The listing builds one solid part. Answer for the finished solid, in the listing's coordinates (mm). Face numbers are marked on the shaded views. A direction names the side the tool comes from. Round coordinates to 2 decimals unless told otherwise and drop trailing zeros. Write each loop counter-clockwise with the first axis right and the second up, starting at its lowest first coordinate (ties: lowest second). Pieces come first, ordered by that corner, then holes.
Item 1: A tool of negligible diameter and unlimited length cuts with its end or side. For the marked faces 1, 2 and 3, from which of +Z, -Z, +X, -X, +Y, -Y can it reach the whole face along a straight path? Write none if from no direction.
Item 2: Find section C-C on y = 6.75. Give the vertices of the cut face in (x, z).
Item 3: Find section B-B on z = -14.75. Give the vertices of the cut face in (x, y).
Item 4: This flat-tipped pin is pushed along its axis until it touches: pin 1 (0.5 mm diameter, centred on x = 0, y = 6.5, fed in from +Z). Where does it stop, or does it pass through?
Item 5: Find section A-A on x = -3. Give the vertices of the cut face in (y, z), then the cut area to 3 significant figures.
Item 6: Find the intervals of material crossed by probe 1 along X at (y, z) = (7, -16); probe 2 along Z at (x, y) = (2, 6.3); probe 3 along Z at (x, y) = (-3, 5.8), in increasing order.
Item 7: Find section D-D on x = -0.25. Give the vertices of the cut face in (y, z), then the cut area to 3 significant figures.
```python
from build123d import *

# Parameters (mm, degrees)
SKETCH1_W           = 80
SKETCH1_H           = 80
SKETCH1_R           = 5
SKETCH1_W_2         = 50
SKETCH1_H_2         = 20
BOSS_EXTRUDE2_DEPTH = 3
BOSS_EXTRUDE3_DEPTH = 20
SCALE2_SCALE        = 0.1


with BuildPart() as part:
    # Sketch1 → Boss-Extrude2 (new body)
    # profile 1 of 2: a face of its own
    with BuildSketch(Plane(origin=(0, 0, 0), x_dir=(1, 0, 0), z_dir=(0, 1, 0))):
        Rectangle(SKETCH1_W, SKETCH1_H)
        with Locations(Location((-30, 30, 0), (0, 0, 90))):
            Circle(SKETCH1_R, mode=Mode.SUBTRACT)
        with Locations(Location((30, 30, 0), (0, 0, 90))):
            Circle(SKETCH1_R, mode=Mode.SUBTRACT)
    # profile 2 of 2: a face of its own
    with BuildSketch(Plane(origin=(0, 0, 0), x_dir=(1, 0, 0), z_dir=(0, 1, 0))):
        with Locations((0, 30)):
            Rectangle(SKETCH1_W_2, SKETCH1_H_2)
    extrude(amount=BOSS_EXTRUDE2_DEPTH)

    # Sketch1_5 → Boss-Extrude3 (add)
    with BuildSketch(Plane(origin=(0, 0, 0), x_dir=(1, 0, 0), z_dir=(0, 1, 0))):
        Polygon((25, 40), (-25, 40), (-25, 30), (-25, 20), (25, 20), (25, 30), align=None)
    extrude(amount=BOSS_EXTRUDE3_DEPTH)


with BuildPart() as part_1:
    # Scale2: scaled about (0, 6.258071502, -13.878534205)
    add(part.part.scale(SCALE2_SCALE).moved(Location((0, 5.632264352, -12.490680785))))


solid = part_1.part
```
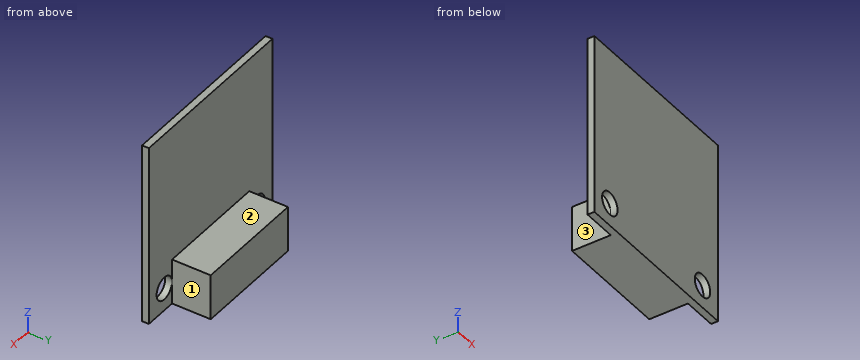
Check values:
1. face 1: +Z, -Z, +X, +Y
1. face 2: +Z, +X, -X, +Y
1. face 3: +Z, -Z, -X, +Y
2. outline: (-2.5, -16.49) - (2.5, -16.49) - (2.5, -14.49) - (-2.5, -14.49) - close
3. outline: (-4, 5.63) - (4, 5.63) - (4, 5.93) - (2.5, 5.93) - (2.5, 7.63) - (-2.5, 7.63) - (-2.5, 5.93) - (-4, 5.93) - close
4. pin 1: stops at z = -14.49
5. outline: (5.63, -16.49) - (5.93, -16.49) - (5.93, -15.99) - (5.63, -15.99) - close; (5.63, -14.99) - (5.93, -14.99) - (5.93, -8.49) - (5.63, -8.49) - close
5. area: 2.10 mm2
6. probe 1: x = -2.5 to 2.5
6. probe 2: z = -16.49 to -14.49
6. probe 3: z = -16.49 to -15.99, -14.99 to -8.49
7. outline: (5.63, -16.49) - (7.63, -16.49) - (7.63, -14.49) - (5.93, -14.49) - (5.93, -8.49) - (5.63, -8.49) - close
7. area: 5.80 mm2
